Input: dimensioned drawing with shaded views. Units: mm. Origin: part minimum x, y, z. Round coordinates to 2 decimals unless told otherwise and drop trailing zeros. Order: outer loops, then holes, each group sorted by start corner. A loop starts at its lowest first (then second) coordinate and runs counter-clockwise, first axis right, second up. Notation, with made-up numbers: (4.25, 53) - (32.25, 53) arc R13 cw to (32.25, 69) - close; hole circle Ø5 at (-32.75, 33.5). An arc over 180 degrees is marked (long way). Put each result on its own line as item: value. Start each with the question number.
(1) Material intervals for L1, parallel to X at y = 21.25, z = 28.75; L2, parallel to Z at x = 545, y = 12.25; L3, parallel to X at y = 27, z = 16.75, sorted ascending. Write a range as [from, to].
(2) Pin query (flat end, axial travel): P1, Ø10, axis at x = 336, z = 5.5, coming from the -Y side; P2, Ø3, axis at x = 225.5, y = 11.5, coming from the -Z side; P3, Ø10, axis at x = 297.5, z = 18.5, coming from the -Y side; P4, Ø18, axis at x = 545, z = 15, coming from the +Y side. Return the tip coordinate at first contact, or that it passes through.
(3) Section C-C (y = 15). Output: boundary loops of the cut face in (x, z).
(4) Section D-D (x = 389). Output: boundary loops of the cut face in (y, z), and give its area (3 significant figures).
(5) Section A-A (z = 15). Output: boundary loops of the cut face in (x, y).
(6) Section B-B (x = 545). Output: boundary loops of the cut face in (y, z).
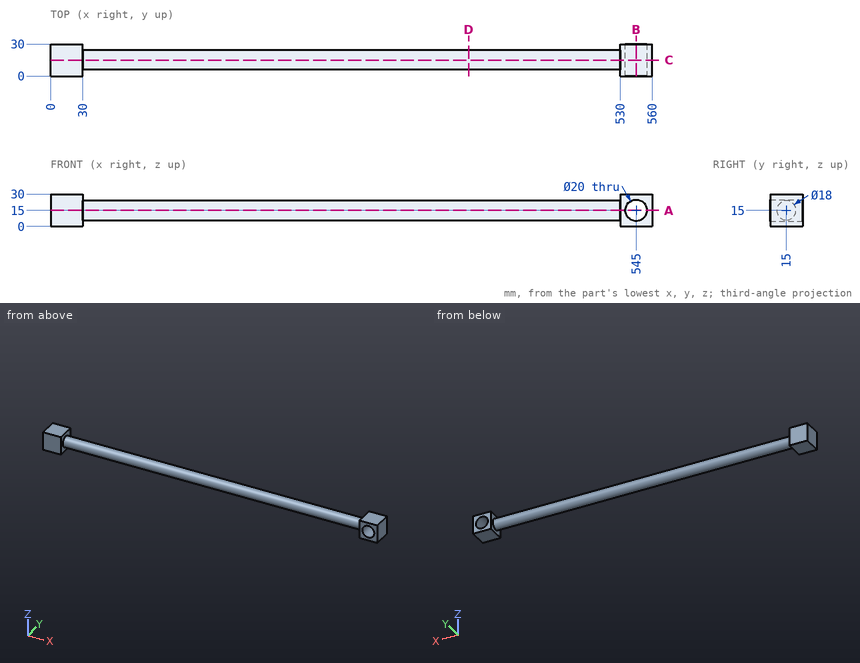
Checks:
1. L1: x = [0, 30], [530, 560]
1. L2: z = [0, 5], [25, 30]
1. L3: x = [0, 30], [530, 535.15], [554.85, 560]
2. P1: stops at y = 7.21
2. P2: stops at z = 6.23
2. P3: stops at y = 6
2. P4: passes through
3. outline: (0, 0) - (30, 0) - (30, 6) - (530, 6) - (530, 0) - (560, 0) - (560, 30) - (530, 30) - (530, 24) - (30, 24) - (30, 30) - (0, 30) - close; hole circle Ø20 at (545, 15)
4. outline: circle Ø18 at (15, 15)
4. area: 254 mm²
5. outline: (0, 0) - (30, 0) - (30, 6) - (530, 6) - (530, 0) - (535, 0) - (535, 30) - (530, 30) - (530, 24) - (30, 24) - (30, 30) - (0, 30) - close; (555, 0) - (560, 0) - (560, 30) - (555, 30) - close
6. outline: (0, 0) - (30, 0) - (30, 5) - (0, 5) - close; (0, 25) - (30, 25) - (30, 30) - (0, 30) - close
